Could you check a few things on this model? Use its own coordinates, in mm. Face numbers are marked on the shaded views. A direction names the side the tool comes from. Give positions to 0.01 mm unless a question says otherwise; leave off trailing zeros. Write each loop counter-clockwise with the first axis right and the second up, starting at its lowest first coordinate (ties: lowest second). Pieces come first, ordered by that corner, then holes. Notation, with made-up numbers: M 16,2 L 73,2 A11 ccw 73,9 Z; hole C 4,46 d9. An arc over 180 degrees is marked long. One line per item, written item: value.
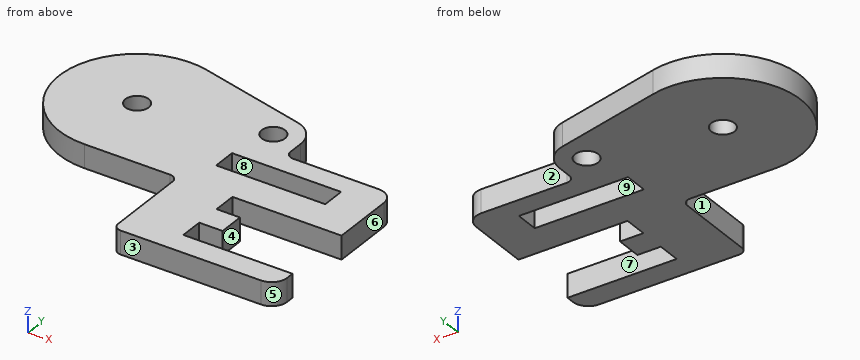
```python
from build123d import *

# Parameters (mm, degrees)
BOSS_EXTRUDE1_DEPTH = 3
SKETCH2_R           = 1.5
CUT_EXTRUDE1_DEPTH  = 3
SKETCH3_W           = 14
SKETCH3_H           = 3
CUT_EXTRUDE2_DEPTH  = 3
SKETCH6_R           = 1.5
CUT_EXTRUDE5_DEPTH  = 3
SKETCH7_W           = 11
SKETCH7_H           = 3.3
CUT_EXTRUDE6_DEPTH  = 3


with BuildPart() as part:
    # Sketch1 → Boss-Extrude1 (new body)
    with BuildSketch(Plane.XY):
        with BuildLine():
            Line((3.822175283, -5.149900319), (3.822175283, -23.449900319))
            ThreePointArc((3.822175283, -23.449900319), (3.236388845, -24.864113882), (1.822175283, -25.449900319))
            Line((1.822175283, -25.449900319), (-16.177824717, -25.449900319))
            ThreePointArc((-16.177824717, -25.449900319), (-16.884931499, -25.157007101), (-17.177824717, -24.449900319))
            Line((-17.177824717, -24.449900319), (-17.177824717, -14.149900319))
            ThreePointArc((-17.177824717, -14.149900319), (-17.470717936, -13.442793538), (-18.177824717, -13.149900319))
            Line((-18.177824717, -13.149900319), (-29.177824717, -13.149900319))
            ThreePointArc((-29.177824717, -13.149900319), (-39.106770847, -1.959930257), (-26.814794989, 6.566893931))
            Line((-26.814794989, 6.566893931), (-12.850764313, 3.170977668))
            ThreePointArc((-12.850764313, 3.170977668), (-10.926033354, 1.932885914), (-10.177824717, -0.229900319))
            Line((-10.177824717, -0.229900319), (-10.177824717, -2.149900319))
            ThreePointArc((-10.177824717, -2.149900319), (-9.884931499, -2.857007101), (-9.177824717, -3.149900319))
            Line((-9.177824717, -3.149900319), (1.822175283, -3.149900319))
            ThreePointArc((1.822175283, -3.149900319), (3.236388845, -3.735686757), (3.822175283, -5.149900319))
        make_face()
    extrude(amount=BOSS_EXTRUDE1_DEPTH)

    # Sketch2 → Cut-Extrude1 (cut)
    with BuildSketch(Plane.XY.offset(3)):
        with Locations((-29.177824717, -3.149900319)):
            Circle(SKETCH2_R)
    extrude(amount=-CUT_EXTRUDE1_DEPTH, mode=Mode.SUBTRACT)

    # Sketch3 → Cut-Extrude2 (cut)
    with BuildSketch(Plane.XY.offset(3)):
        with Locations((-8.177824717, -7.349900319)):
            Rectangle(SKETCH3_W, SKETCH3_H)
        with Locations((-3.177824717, -14.649900319)):
            Rectangle(SKETCH3_W, SKETCH3_H)
        with Locations((-3.177824717, -20.949900319)):
            Rectangle(SKETCH3_W, SKETCH3_H)
    extrude(amount=-CUT_EXTRUDE2_DEPTH, mode=Mode.SUBTRACT)

    # Sketch6 → Cut-Extrude5 (cut)
    with BuildSketch(Plane.XY.offset(3)):
        with Locations((-13.677824717, -0.229900319)):
            Circle(SKETCH6_R)
    extrude(amount=-CUT_EXTRUDE5_DEPTH, mode=Mode.SUBTRACT)

    # Sketch7 → Cut-Extrude6 (cut)
    with BuildSketch(Plane.XY.offset(3)):
        with Locations((-1.677824717, -17.799900319)):
            Rectangle(SKETCH7_W, SKETCH7_H)
    extrude(amount=-CUT_EXTRUDE6_DEPTH, mode=Mode.SUBTRACT)


solid = part.part
```
1) If we section it at C-C, the plane y = 0.5: Write out the boundary of the cut face in (x, z), then the cut area to 3 significant figures.
Outcome:
outline: M -38.49,0 L -14.99,0 L -14.99,3 L -38.49,3 Z; M -12.37,0 L -10.25,0 L -10.25,3 L -12.37,3 Z
area: 76.8 mm^2
2) On a 3-axis mill with a long thin cutter (end or side, diameter ignored), from which of +Z, -Z, +X, -X, +Y, -Y can I reach the whole of each face in a straight line? I mean the marked faces 1, 2, 3, 4 and 5. Say none if no direction works.
Outcome:
face 1: +Z, -Z, -X, -Y
face 2: +Z, -Z, +X, +Y
face 3: +Z, -Z, +X, -X, -Y
face 4: +Z, -Z, +X
face 5: +Z, -Z, +X, -Y
3) Please list where these lines run through material, in increasing order: L1, parallel to Y at x = -1.5, z = 1.2; L2, parallel to Y at x = -8.5, z = 2.2; L3, parallel to X at y = -15, z = 0.3. Write a range as from..to.
Outcome:
L1: y = -25.45..-22.45, -13.15..-8.85, -5.85..-3.15
L2: y = -25.45..-22.45, -19.45..-16.15, -13.15..-8.85, -5.85..-3.15
L3: x = -17.18..-10.18
4) If we section it at A-A, the plane x = -2: Write out the boundary of the cut face in (y, z), then the cut area to 3 significant figures.
Outcome:
outline: M -25.45,0 L -22.45,0 L -22.45,3 L -25.45,3 Z; M -13.15,0 L -8.85,0 L -8.85,3 L -13.15,3 Z; M -5.85,0 L -3.15,0 L -3.15,3 L -5.85,3 Z
area: 30.0 mm^2
5) We'd pull the mould along X, two halves only. Please class the marked faces 6, 7, 8 and 9: pulls with the +X half, pulls with the -X half, needs draft (parallel to the pull), parting line crosses it, or undercut.
Outcome:
face 6: pulls with the +X half
face 7: needs draft
face 8: undercut
face 9: undercut
6) I'm going to push flat-ended pins straight in: pin 1 (0.9 mm diameter, centred on x = -11, z = 1, fed in from +Y); pin 2 (0.9 mm diameter, centred on x = 0, z = 2, fed in from +Y); pin 3 (1.5 mm diameter, centred on y = -1, z = 2, fed in from +X). Where does each tip first touch, or does it pass through?
Outcome:
pin 1: stops at y = 2.47
pin 2: stops at y = -3.15
pin 3: stops at x = -10.18
7) If we section it at D-D, the plane x = -8: Write out the boundary of the cut face in (y, z), then the cut area to 3 significant figures.
Outcome:
outline: M -25.45,0 L -22.45,0 L -22.45,3 L -25.45,3 Z; M -19.45,0 L -16.15,0 L -16.15,3 L -19.45,3 Z; M -13.15,0 L -8.85,0 L -8.85,3 L -13.15,3 Z; M -5.85,0 L -3.15,0 L -3.15,3 L -5.85,3 Z
area: 39.9 mm^2
8) If we section it at B-B, the plane z = 1.25: Write out the boundary of the cut face in (x, y).
Outcome:
outline: M -29.18,-13.15 L -18.18,-13.15 A1 cw -17.18,-14.15 L -17.18,-24.45 A1 ccw -16.18,-25.45 L 1.82,-25.45 A2 ccw 3.82,-23.45 L 3.82,-22.45 L -10.18,-22.45 L -10.18,-19.45 L -7.18,-19.45 L -7.18,-16.15 L -10.18,-16.15 L -10.18,-13.15 L 3.82,-13.15 L 3.82,-5.15 A2 ccw 1.82,-3.15 L -9.18,-3.15 A1 cw -10.18,-2.15 L -10.18,-0.23 A3.5 ccw -12.85,3.17 L -26.81,6.57 A10 ccw long Z; hole C -29.18,-3.15 d3; hole M -15.18,-8.85 L -1.18,-8.85 L -1.18,-5.85 L -15.18,-5.85 Z; hole C -13.68,-0.23 d3
